Build history of the part. All positions in model axes, mm. A direction names the side the tool comes from. Coordinates: 2 decimals unless noted, no trailing zeros. Order: outer loops, then holes, each group sorted by start corner. A loop starts at its lowest first (then second) coordinate and runs counter-clockwise, first axis right, second up. Notation, with made-up numbers: M 73,20 L 109,20 A24 ccw 109,32 Z; hole C 18,16 d7. An arc over 180 degrees is marked long. Write item = value, one per line. Start each with the question number.
Q1. Pin check, flat tips, straight feed: P1, Ø5, axis at x = -436.5, z = -16.5, coming from the +Y side; P2, Ø6, axis at x = -300.04, z = -11.11, coming from the -Y side (3 decimals); P3, Ø1.5, axis at x = -159.5, y = 6, coming from the +Z side (3 decimals); P4, Ø12, axis at x = -456, y = 5.5, coming from the +Z side. Stop position of each tip, or through.
Q2. Band-saw the part on B-B on y = 10.75. Write the cut outline in (x, z) (3 decimals).
Q3. 3-axis set-ups, long thin cutter, end or side, ignore diameter. For faces 1 (the face through (-277, 11, -22.225)), 2 (the face through (-277, -3.175, -13)): which of +Z, -Z, +X, -X, +Y, -Y reach the whole face in a straight line?
Q4. Drill centre lines: probe 1 along Z at (x, y) = (-484, 7) (3 decimals); probe 2 along Y at (x, z) = (-224.5, -15) (3 decimals); probe 3 along Y at (x, z) = (-381, -2.5) (3 decimals). Where is each one in solid material? Low to high.
Q5. Band-saw the part on A-A on x = -144. Write the cut outline in (y, z) (3 decimals).
```python
from build123d import *

# Parameters (mm, degrees)
F1_DEPTH = 561.975
F2_R     = 2.6162
F3_DEPTH = 25.4


with BuildPart() as f1:
    # F0 (on Right) → F1 (new body)
    with BuildSketch(Plane.YZ):
        with BuildLine():
            Line((0, -19.05), (0, -3.175))
            ThreePointArc((0, -3.175), (-0.929936, -0.929936), (-3.175, 0))
            Line((-3.175, 0), (-3.175, -25.4))
            Line((-3.175, -25.4), (22.225, -25.4))
            ThreePointArc((22.225, -25.4), (21.295064, -23.154936), (19.05, -22.225))
            Line((19.05, -22.225), (3.175, -22.225))
            ThreePointArc((3.175, -22.225), (0.929936, -21.295064), (0, -19.05))
        make_face()
    extrude(amount=-F1_DEPTH)

    # F2 (on face) → F3 (cut)
    with BuildSketch(Plane(origin=(0, 0, 0), x_dir=(-1, 0, 0), z_dir=(0, 1, 0))):
        with Locations((10.31875, -11.1125)):
            Circle(F2_R)
        with Locations((280.9875, -11.1125)):
            Circle(F2_R)
        with Locations((551.6626, -11.1125)):
            Circle(F2_R)
        with Locations((128.5875, -11.1125)):
            Circle(F2_R)
        with Locations((204.7875, -11.1125)):
            Circle(F2_R)
        with Locations((357.1875, -11.1125)):
            Circle(F2_R)
        with Locations((433.3875, -11.1125)):
            Circle(F2_R)
        with Locations((509.5875, -11.1125)):
            Circle(F2_R)
        with Locations((52.3875, -11.1125)):
            Circle(F2_R)
        with Locations((261.9375, -11.1125)):
            Circle(F2_R)
        with Locations((300.0375, -11.1125)):
            Circle(F2_R)
    extrude(amount=-F3_DEPTH, mode=Mode.SUBTRACT)


solid = f1.part
```
Recorded:
q1.P1 = 0
q1.P2 = -3.175
q1.P3 = -22.225
q1.P4 = -1.46
q2.outline = M -561.975,-25.4 L 0,-25.4 L 0,-22.225 L -561.975,-22.225 Z
q3.face_1 = +Z, +X, -X, +Y
q3.face_2 = +Z, -Z, +X, -X, -Y
q4.probe_1 = -25.4 to -22.225
q4.probe_2 = -3.175 to 0
q4.probe_3 = -3.175 to -0.073
q5.outline = M -3.175,-25.4 L 22.225,-25.4 A3.175 ccw 19.05,-22.225 L 3.175,-22.225 A3.175 cw 0,-19.05 L 0,-3.175 A3.175 ccw -3.175,0 Z
